Input: part model. Units: mm. Frame: model coordinates. Face numbers are marked on the shaded views. A direction names the side the tool comes from. Coordinates: 2 decimals unless noted, no trailing zeros. Loops run counter-clockwise (first coordinate to the right, second up) from the corner with the lowest first, then second, coordinate; pieces in that order, holes last.
Item 1: Section B-B on z = -151. Return loops of the section in (x, y), and give its area (3 significant figures).
Item 2: Contact query for flat-ended pins moving along their axis: P1, Ø1.3, axis at x = 303, z = 353.5, coming from the +Y side; P2, Ø8, axis at y = 321.5, z = -251.5, coming from the +X side; P3, Ø0.5, axis at x = 303, z = -351.5, coming from the +Y side; P4, Ø3, axis at y = 4.5, z = 7.5, coming from the +X side. Output: stop coordinate, or through.
Item 3: Pull-direction query (Z, two-part tool) for the marked faces 1, 2, 3 and 4; classes: released by +Z, released by -Z, zero draft, split by the parting line, or undercut.
Item 4: Reachability of the marked faces 5 and 6 from +Z, -Z, +X, -X, +Y, -Y: full face, straight path, thin tool, end or side. Return the list, or none.
Item 5: Section C-C on x = -188. Return loops of the section in (y, z).
Item 6: Section A-A on y = 428. Return loops of the section in (x, z), and give its area (3 significant figures).
Item 7: Ray query, line 1 along Y through (x, z) = (118, -139); line 2 along Z through (x, y) = (-233.5, 545.5); line 3 along X through (y, z) = (89.5, 201). Return the intervals inside material, ascending.
```python
from build123d import *

# Parameters (mm, degrees)
SKETCH1_W            = 604.8
SKETCH1_H            = 711.2
BOSS_EXTRUDE1_DEPTH  = 812.8
SKETCH2_W            = 700
SKETCH2_H            = 800
BOSS_EXTRUDE2_DEPTH  = 600
SKETCH2_2_W          = 700
SKETCH2_2_H          = 800
CUT_EXTRUDE1_DEPTH   = 600
SKETCH3_W            = 5.6
SKETCH3_H            = 6.4
BOSS_EXTRUDE3_DEPTH  = 4.8
FILLET1_R            = 3.2
SKETCH4_R            = 1
BOSS_EXTRUDE4_DEPTH  = 10
FILLET1_OF_MIRROR1_R = 3.2


with BuildPart() as part:
    # Sketch1 → Boss-Extrude1 (new body)
    with BuildSketch(Plane(origin=(0, 0, 0), x_dir=(1, 0, 0), z_dir=(0, 1, 0))):
        Rectangle(SKETCH1_W, SKETCH1_H)
    extrude(amount=BOSS_EXTRUDE1_DEPTH)

    # Sketch2 → Boss-Extrude2 (add)
    with BuildSketch(Plane(origin=(302.4, 0, 0), x_dir=(0, 0, -1), z_dir=(1, 0, 0))):
        with Locations((0, 406.4)):
            Rectangle(SKETCH2_W, SKETCH2_H)
    extrude(amount=-BOSS_EXTRUDE2_DEPTH)

    # Sketch2<2> → Cut-Extrude1 (cut)
    with BuildSketch(Plane(origin=(302.4, 0, 0), x_dir=(0, 0, -1), z_dir=(1, 0, 0))):
        with Locations((0, 406.4)):
            Rectangle(SKETCH2_2_W, SKETCH2_2_H)
    extrude(amount=-CUT_EXTRUDE1_DEPTH, mode=Mode.SUBTRACT)

    # Sketch3 → Boss-Extrude3 (add)
    with BuildSketch(Plane(origin=(302.4, 0, 0), x_dir=(0, 0, -1), z_dir=(1, 0, 0))):
        with Locations((-352.8, 3.2)):
            Rectangle(SKETCH3_W, SKETCH3_H)
    boss_extrude3 = extrude(amount=BOSS_EXTRUDE3_DEPTH)

    # Fillet1
    fillet1_edges = [part.edges().sort_by_distance(p)[0] for p in [
        (307.2, 0, 352.8),
        (307.2, 6.4, 352.8),
    ]]
    fillet(fillet1_edges, radius=FILLET1_R - 0.0001)  # a hair under: the kernel refuses the full size

    # Sketch4 → Boss-Extrude4 (add)
    with BuildSketch(Plane(origin=(0, 0, 350), x_dir=(-1, 0, 0), z_dir=(0, 0, -1))):
        with Locations(Location((-304.8, 3.2, 0), (0, 0, 180))):
            Circle(SKETCH4_R)
    boss_extrude4 = extrude(amount=BOSS_EXTRUDE4_DEPTH)

    # Mirror1: Boss-Extrude3, Boss-Extrude4 across plane
    add(boss_extrude3.mirror(Plane.XY))
    add(boss_extrude4.mirror(Plane.XY))

    # Fillet1 of Mirror1
    fillet1_of_mirror1_edges = [part.edges().sort_by_distance(p)[0] for p in [
        (307.2, 0, -352.8),
        (307.2, 6.4, -352.8),
    ]]
    fillet(fillet1_of_mirror1_edges, radius=FILLET1_OF_MIRROR1_R - 0.0001)  # a hair under: the kernel refuses the full size


solid = part.part
```
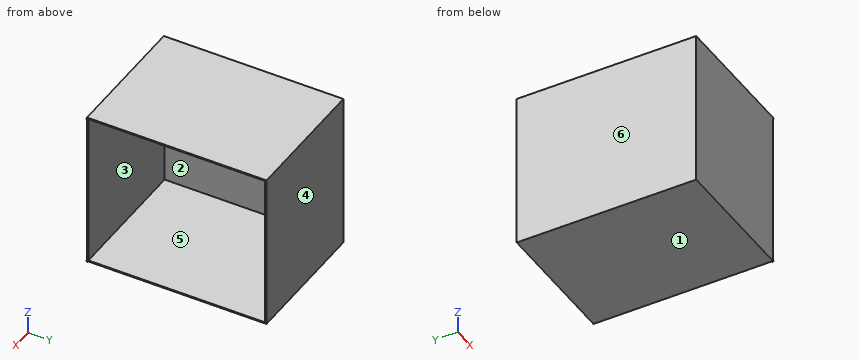
Results found:
1. outline: (-302.4, 0) - (302.4, 0) - (302.4, 6.4) - (-297.6, 6.4) - (-297.6, 806.4) - (302.4, 806.4) - (302.4, 812.8) - (-302.4, 812.8) - close
1. area: 11,600 mm2
2. P1: stops at y = 812.8
2. P2: stops at x = -297.6
2. P3: stops at y = 6.4
2. P4: stops at x = 302.4
3. face 1: released by -Z
3. face 2: undercut
3. face 3: undercut
3. face 4: zero draft
4. face 5: +X
4. face 6: +Z, -Z, -X, +Y, -Y
5. outline: (0, -355.6) - (812.8, -355.6) - (812.8, 355.6) - (0, 355.6) - close; hole (6.4, -350) - (806.4, -350) - (806.4, 350) - (6.4, 350) - close
6. outline: (-302.4, -355.6) - (302.4, -355.6) - (302.4, -350) - (-297.6, -350) - (-297.6, 350) - (302.4, 350) - (302.4, 355.6) - (-302.4, 355.6) - close
6. area: 10,100 mm2
7. line 1: y = 0 to 6.4, 806.4 to 812.8
7. line 2: z = -355.6 to -350, 350 to 355.6
7. line 3: x = -302.4 to -297.6
